Design review of the part built by this model. Coordinates are the model's own, in mm. A direction names the side the tool comes from. Coordinates: 2 decimals unless noted, no trailing zeros. Loops run counter-clockwise (first coordinate to the right, second up) from the corner with the lowest first, then second, coordinate; pieces in that order, holes last. Notation, with made-up numbers: M 55,-12.75 L 97,-12.75 A21 cw 97,-4.75 Z; hole C 80,76 d4. An arc over 180 degrees is marked long. Answer as a JSON object with one key per item and string values. Group by question number.
1. To check wall thickness, follow probe 1 along Z at (x, y) = (20.25, 0.8); probe 2 along X at (y, z) = (3.6, 2.5); probe 3 along Y at (x, z) = (-18, 11) (3 decimals). State the ranges of each line that lie inside material, in increasing order.
2. Machinability: for faces 1 (the flat face through (-14, 3.46, 6)), 2 (the cylindrical face through (-4.5, 0.9, 5.9)), 3 (the flat face through (-9.7, 3.9, 5.5)), 4 (the flat face through (8, 2.5, 3)), 5 (the flat face through (-9.7, 3.9, 1.5)), which of the approach directions +Z, -Z, +X, -X, +Y, -Y give a long, thin tool a straight path to every point of the face, cutting with its end or side? Answer none if there is none.
3. Consider section B-B (x = 13.5). State the section outline as (y, z) points (3 decimals), then the cut area to 3 significant figures.
4. Consider section A-A (x = 20.25). State the section outline as (y, z) points (3 decimals), then the cut area to 3 significant figures.
5. Consider section C-C (x = 3.5). State the section outline as (y, z) points.
6. Insertion check: pin 1 (0.6 mm diameter, centred on x = 25, z = 2.5, fed in from -Y); pin 2 (0.8 mm diameter, centred on x = -10, y = 4, fed in from +Z); pin 3 (2 mm diameter, centred on x = 13, y = 1.5, fed in from -Z); pin 4 (0.5 mm diameter, centred on x = -18.5, y = 4, fed in from -Z). Each pin has a flat end and moves straight along its axis. Give the tip position at first contact, or say it passes through.
Autodesk Inventor part; units mm, degrees
ref_plane "Work Plane1" through (-2.9282, 3.7996, 12.5) normal (0, 1, 0) x (1, 0, 0)
ref_plane "Work Plane2" through (0, 0, 1.5) normal (0, 0, -1) x (-1, 0, 0)
ref_plane "Work Plane4" through (0, 0, 0.45) normal (0, 0, -1) x (-1, 0, 0)
sketch "Sketch1" plane through (0, 0, 0) normal (0, 0, 1) x (1, 0, 0)
  arc A0 (-21.6, 0) -> (-23.4, 0) centre (-22.5, 0) ccw
  arc A1 (-15.975, 0) -> (-20.025, 0) centre (-18, 0) ccw
  arc A2 (-11.475, 0) -> (-15.525, 0) centre (-13.5, 0) ccw
  arc A3 (-6.975, 0) -> (-11.025, 0) centre (-9, 0) ccw
  arc A4 (-3.6, 0) -> (-5.4, 0) centre (-4.5, 0) ccw
  arc A5 (2.025, 0) -> (-2.025, 0) centre (0, 0) ccw
  arc A6 (6.525, 0) -> (2.475, 0) centre (4.5, 0) ccw
  arc A7 (11.025, 0) -> (6.975, 0) centre (9, 0) ccw
  arc A8 (15.525, 0) -> (11.475, 0) centre (13.5, 0) ccw
  arc A9 (18.875, 0) -> (17.125, 0) centre (18, 0) ccw
  arc A10 (23.375, 0) -> (21.625, 0) centre (22.5, 0) ccw
  line L0 (-25, 0) -> (-25, 1.5)
  line L1 (-25, 0) -> (25, 0)
  line L2 (25, 0) -> (25, 1.5)
  arc A11 (25, 1.5) -> (24, 2.5) centre (24, 1.5) ccw
  arc A12 (-24, 2.5) -> (-25, 1.5) centre (-24, 1.5) ccw
  line L3 (-8.467, 2.5) -> (24, 2.5)
  line L4 (-19.1661, 2.65) -> (-18.6985, 3.46)
  line L5 (-18.6985, 3.46) -> (-9.1945, 3.46)
  line L6 (-9.1945, 3.46) -> (-8.7268, 2.65)
  line L7 (-9.1945, 3.46) -> (-8.2592, 3.46) construction
  arc A13 (-8.7268, 2.65) -> (-8.467, 2.5) centre (-8.467, 2.8) ccw
  line L8 (-19.4259, 2.5) -> (-24, 2.5)
  arc A14 (-19.4259, 2.5) -> (-19.1661, 2.65) centre (-19.4259, 2.8) ccw
  line L9 (0, 0) -> (0, 12.7088) construction
  point P0 (-19.2527, 2.5)
  point P1 (-8.6402, 2.5)
  dimension "d1" = 1.8
  dimension "d2" = 4.5
  dimension "d3" = 4.5
  dimension "d4" = 4.5
  dimension "d5" = 4.5
  dimension "d6" = 4.5
  dimension "d7" = 4.5
  dimension "d8" = 4.5
  dimension "d9" = 4.5
  dimension "d10" = 4.5
  dimension "d11" = 4.5
  dimension "d12" = 4.05
  dimension "d13" = 4.05
  dimension "d14" = 4.05
  dimension "d15" = 1.8
  dimension "d16" = 4.05
  dimension "d17" = 4.05
  dimension "d18" = 4.05
  dimension "d19" = 4.05
  dimension "d20" = 1.75
  dimension "d21" = 1.75
  dimension "d22" = 2.5
  dimension "d23" = 50
  dimension "d24" = 1.5
  dimension "d25" = 1.5
  dimension "d26" = 1
  dimension "d27" = 1
  dimension "d29" = 120
  dimension "d32" = 9.504
  dimension "d33" = 60
  dimension "d67" = 0.96
  dimension "d68" = 0.3
  dimension "d69" = 0.3
  dimension "d70" = 33.467
  dimension "d71" = 5.5741
extrude "Extrusion1" add sketch "Sketch1" along normal blind 12 contours A0 L1 L0 A12 L8 A14 L4 L5 L6 A13 L3 A11 L2 A10 A9 A8 A7 A6 A5 A4 A3 A2 A1
sketch "Sketch2" plane through (0, 0, 12) normal (0, 0, 1) x (1, 0, 0)
  line L0 (-9.1945, 3.46) -> (-18.6985, 3.46)
  point P0 (0, 0)
  point P1 (-16.1965, 3.46)
  point P2 (-11.6965, 3.46)
  dimension "d39" = 4.5
  dimension "d40" = 2.502
hole "Hole1" at (-16.1965, 3.46, 12) at (-11.6965, 3.46, 12) direction (0, 0, -1) diameter 2 end through all
sketch "Sketch3" plane through (24, 2.5, 12) normal (0, 1, 0) x (1, 0, 0)
  line L0 (0.714, 6.4) -> (-32.467, 6.4)
  line L1 (-32.467, 6.4) -> (-32.467, 7)
  line L2 (-32.467, 7) -> (0.714, 7)
  line L3 (0.714, 7) -> (0.714, 6.4)
  line L4 (-32.467, 11) -> (0.714, 11)
  line L5 (0.714, 11) -> (0.714, 11.6)
  line L6 (0.714, 11.6) -> (-32.467, 11.6)
  line L7 (-32.467, 11.6) -> (-32.467, 11)
  line L8 (1, 12) -> (1, 0)
  line L9 (0, 12) -> (-32.467, 12)
  line L10 (-43.4259, 6.4) -> (-48.29, 6.4)
  line L11 (-48.29, 6.4) -> (-48.29, 7)
  line L12 (-48.29, 7) -> (-43.4259, 7)
  line L13 (-43.4259, 7) -> (-43.4259, 6.4)
  line L14 (-43.4259, 11.6) -> (-48.29, 11.6)
  line L15 (-48.29, 11.6) -> (-48.29, 11)
  line L16 (-48.29, 11) -> (-43.4259, 11)
  line L17 (-43.4259, 11) -> (-43.4259, 11.6)
  line L18 (-49, 12) -> (-49, 0)
  point P0 (-24, 12)
  point P1 (-32.5535, 12.5)
  point P2 (-32.467, 12)
  point P3 (-43.4259, 12)
  dimension "d48" = 0.286
  dimension "d49" = 0.286
  dimension "d50" = 0.6
  dimension "d51" = 0.6
  dimension "d57" = 0.4
  dimension "d58" = 4
  dimension "d79" = 0.71
extrude "Extrusion2" cut sketch "Sketch3" against normal blind 0.3
ref_plane "Work Plane1" through (-2.9282, 3.7996, 12.5) normal (0, 1, 0) x (1, 0, 0)
sketch "Sketch4" plane through (-2.9282, 2.5, 12.5) normal (0, 1, 0) x (1, 0, 0)
  line L0 (27.9282, 12.5495) -> (27.9282, 3.2148)
  line L1 (26.9282, 11.5) -> (-5.5388, 11.5)
  line L2 (27.9282, 12.5) -> (27.9282, 0.5)
  line L3 (-22.0718, 12.5) -> (-22.0718, 0.5)
  point P0 (2.9282, 12.5)
  point P1 (-17.8838, 9.5)
  point P2 (0.1157, 9.5)
  point P3 (23.1782, 9.5)
  dimension "d54" = 4.75
  dimension "d72" = 2
  dimension "d121" = 4.188
  dimension "d122" = 23.0625
hole "Hole2" at (-20.812, 2.5, 3) at (-2.8125, 2.5, 3) at (20.25, 2.5, 3) direction (0, -1, 0) diameter 1.5 end through all both
sketch "Sketch5" plane through (-8.467, 2.5, 12) normal (0, 1, 0) x (1, 0, 0)
  circle A0 centre (34.867, 2.0003) radius 2
  line L0 (32.467, 0) -> (33.467, 0)
  line L1 (33.467, 12) -> (33.467, 0)
  line L2 (33.467, 0) -> (33.467, 0.572)
  point P0 (8.467, 12)
  dimension "d73" = 4
  dimension "d75" = 1.4
  dimension "d76" = 0.572
extrude "Extrusion3" cut sketch "Sketch5" against normal blind 7.05
mirror "Mirror1" about plane through (0, 0, 0) normal (1, 0, 0) of "Extrusion3"
ref_plane "Work Plane2" through (0, 0, 1.5) normal (0, 0, -1) x (-1, 0, 0)
sketch "Sketch6" plane through (0, 0, 1.5) normal (0, 0, -1) x (-1, 0, 0)
  line L0 (8.7268, 2.65) -> (9.1945, 3.46)
  line L1 (9.1945, 3.46) -> (9.7718, 4.46)
  line L2 (9.1945, 3.46) -> (10.6965, 3.46)
  line L3 (9.7718, 4.46) -> (9.9768, 4.46)
  line L4 (9.9768, 4.46) -> (10.1968, 4.16)
  line L5 (10.1968, 4.16) -> (9.8968, 4.16)
  line L6 (9.8968, 4.16) -> (9.8968, 3.46)
  line L7 (9.1945, 3.46) -> (10.6965, 3.46)
  line L8 (9.8968, 3.46) -> (9.1945, 3.46)
  line L9 (12.6965, 3.46) -> (15.1965, 3.46)
  line L10 (13.9465, 3.46) -> (13.9465, 5.3261) construction
  line L11 (17.1965, 3.46) -> (18.6985, 3.46)
  line L12 (18.6985, 3.46) -> (18.1211, 4.46)
  line L13 (18.6985, 3.46) -> (19.8532, 3.46) construction
  line L14 (18.1211, 4.46) -> (17.9161, 4.46)
  line L15 (17.9161, 4.46) -> (17.6961, 4.16)
  line L16 (17.6961, 4.16) -> (17.9961, 4.16)
  line L17 (17.9961, 4.16) -> (17.9961, 3.46)
  line L18 (17.9961, 3.46) -> (18.6985, 3.46)
  point P0 (0, 0)
  dimension "d81" = 1
  dimension "d82" = 0.205
  dimension "d83" = 126.25
  dimension "d84" = 0.3
  dimension "d85" = 0.3
  dimension "d94" = 120
  dimension "d95" = 1
  dimension "d96" = 0.205
  dimension "d97" = 53.75
  dimension "d98" = 53.75
  dimension "d99" = 0.3
  dimension "d100" = 0.3
extrude "Extrusion4" add sketch "Sketch6" against normal blind 4
ref_plane "Work Plane4" through (0, 0, 0.45) normal (0, 0, -1) x (-1, 0, 0)
sketch "Sketch7" plane through (0, 0, 0.45) normal (0, 0, -1) x (-1, 0, 0)
  line L0 (24.9987, 1.55) -> (24.4667, 1.55)
  line L1 (25, 0) -> (20.025, 0)
  arc A0 (15.1965, 3.46) -> (17.1965, 3.46) centre (16.1965, 3.46) ccw
  line L2 (12.6965, 3.46) -> (15.1965, 3.46)
  arc A1 (10.6965, 3.46) -> (12.6965, 3.46) centre (11.6965, 3.46) ccw
  line L3 (9.1945, 3.46) -> (10.6965, 3.46)
  line L4 (8.7268, 2.65) -> (9.1945, 3.46)
  arc A2 (8.467, 2.5) -> (8.7268, 2.65) centre (8.467, 2.8) ccw
  line L5 (-24, 2.5) -> (8.467, 2.5)
  arc A3 (-24, 2.5) -> (-25, 1.5) centre (-24, 1.5) ccw
  line L6 (-25, 0) -> (-25, 1.5)
  line L7 (-23.375, 0) -> (-25, 0)
  arc A4 (-21.625, 0) -> (-23.375, 0) centre (-22.5, 0) ccw
  line L8 (-18.875, 0) -> (-21.625, 0)
  arc A5 (-17.125, 0) -> (-18.875, 0) centre (-18, 0) ccw
  line L9 (-15.525, 0) -> (-17.125, 0)
  arc A6 (-11.475, 0) -> (-15.525, 0) centre (-13.5, 0) ccw
  line L10 (-11.025, 0) -> (-11.475, 0)
  arc A7 (-6.975, 0) -> (-11.025, 0) centre (-9, 0) ccw
  line L11 (-6.525, 0) -> (-6.975, 0)
  arc A8 (-2.475, 0) -> (-6.525, 0) centre (-4.5, 0) ccw
  line L12 (-2.025, 0) -> (-2.475, 0)
  arc A9 (2.025, 0) -> (-2.025, 0) centre (0, 0) ccw
  line L13 (3.6, 0) -> (2.025, 0)
  arc A10 (5.4, 0) -> (3.6, 0) centre (4.5, 0) ccw
  line L14 (6.975, 0) -> (5.4, 0)
  arc A11 (11.025, 0) -> (6.975, 0) centre (9, 0) ccw
  line L15 (11.475, 0) -> (11.025, 0)
  arc A12 (15.525, 0) -> (11.475, 0) centre (13.5, 0) ccw
  line L16 (15.975, 0) -> (15.525, 0)
  arc A13 (20.025, 0) -> (15.975, 0) centre (18, 0) ccw
  line L17 (25, 0) -> (23.4, 0)
  line L18 (25, 1.5) -> (25, 0)
  arc A14 (25, 1.5) -> (24, 2.5) centre (24, 1.5) ccw
  line L19 (19.4259, 2.5) -> (24, 2.5)
  arc A15 (19.1661, 2.65) -> (19.4259, 2.5) centre (19.4259, 2.8) ccw
  line L20 (18.6985, 3.46) -> (19.1661, 2.65)
  line L21 (17.1965, 3.46) -> (18.6985, 3.46)
  line L22 (24.4667, 1.55) -> (24.124, 0.7504)
  line L23 (24.4667, 1.55) -> (25.3367, 1.55) construction
  line L24 (24.124, 0.7504) -> (24.4, 0.7504)
  line L25 (24.4, 0.7504) -> (24.4, 0)
  line L26 (24.4, 0) -> (25, 0)
  arc A16 (25, 1.5) -> (24, 2.5) centre (24, 1.5) ccw
  line L27 (25, 0) -> (25, 1.5)
  line L28 (21.6, 0) -> (20.025, 0)
  arc A17 (23.4, 0) -> (21.6, 0) centre (22.5, 0) ccw
  point P0 (0, 0)
  dimension "d102" = 1.55
  dimension "d103" = 0.532
  dimension "d104" = 113.2
  dimension "d105" = 0.87
  dimension "d106" = 0.276
extrude "Extrusion5" cut sketch "Sketch7" against normal blind 6.1 contours A14 L18 L1 L25 L24 L22 L0
sketch "Sketch8" plane through (0, 0, 12) normal (0, 0, 1) x (1, 0, 0)
  line L0 (-22, 0) -> (23, 0)
  line L1 (23, 0) -> (23, 0.175)
  line L2 (23, 0.175) -> (-22, 0.175)
  line L3 (-22, 0.175) -> (-22, 0)
  line L4 (25, 0) -> (25, 1.5)
  point P0 (0, 0)
  point P1 (21.625, 0)
  dimension "d109" = 0.175
  dimension "d110" = 45
  dimension "d111" = 2
extrude "Extrusion6" cut sketch "Sketch8" against normal through all
ref_plane "Work Plane5" through (0, 0, 0.75) normal (0, 0, -1) x (-1, 0, 0)
sketch "Sketch9" plane through (0, 0, 0.75) normal (0, 0, -1) x (-1, 0, 0)
  line L0 (24.9987, 1.55) -> (24.4667, 1.55)
  line L1 (25, 0) -> (24.25, 0)
  line L2 (25, 1.5) -> (25, 0)
  line L3 (24.4667, 1.55) -> (24.124, 0.7504)
  line L4 (24.4667, 1.55) -> (25.3367, 1.55) construction
  line L5 (24.124, 0.7504) -> (24.4, 0.7504)
  line L6 (24.4, 0.7504) -> (24.4, 0)
  line L7 (24.4, 0) -> (25, 0)
  line L8 (25, 0) -> (25, 1.5)
  line L9 (0, 0) -> (0, 5.6827) construction
  line L10 (-24.9987, 1.55) -> (-24.4667, 1.55)
  line L11 (-24.4, 0.7504) -> (-24.4, 0)
  line L12 (-25, 0.7504) -> (-25, 0)
  line L13 (-24.4, 0) -> (-25, 0)
  line L14 (-25, 0) -> (-25, 1.5)
  line L15 (-24.4667, 1.55) -> (-25.3367, 1.55) construction
  line L16 (-25, 0) -> (-24.25, 0)
  line L17 (-24.124, 0.7504) -> (-24.4, 0.7504)
  line L18 (-24.4667, 1.55) -> (-24.124, 0.7504)
  arc A0 (-24, 2.5) -> (-25, 1.5) centre (-24, 1.5) ccw
  arc A1 (-24.9987, 1.55) -> (-25, 1.5) centre (-24, 1.5) ccw
  point P0 (24.25, 0)
  point P1 (24, 1.5)
  point P2 (24, 1.5)
  point P3 (-24.25, 0)
  point P4 (-24, 1.5)
  point P5 (-24, 1.5)
  dimension "d115" = 0.532
  dimension "d116" = 113.2
  dimension "d117" = 0.87
  dimension "d118" = 0.276
extrude "Extrusion7" cut sketch "Sketch9" against normal blind 6.1
properties part number "3d_LM - Pinza 2" material "PA12 SLS 3D Print"
Findings below:
{
 "1": {"probe 1": "z = 0 to 2.25, 3.75 to 12", "probe 2": "x = -18.62 to -18, -9.9 to -9.28", "probe 3": "y = 2.025 to 3.46"},
 "2": {"face 1": "+Z, -Z, +Y", "face 2": "+Z, -Z, -Y", "face 3": "+Z, +X, -X, +Y", "face 4": "+Z, -Z, +X, +Y", "face 5": "-Z, +X, -X, +Y"},
 "3": {"outline": "M 2.025,0 L 2.5,0 L 2.5,0.4 L 2.2,0.4 L 2.2,1 L 2.5,1 L 2.5,5 L 2.2,5 L 2.2,5.6 L 2.5,5.6 L 2.5,12 L 2.025,12 Z", "area": "5.34 mm^2"},
 "4": {"outline": "M 0.175,0 L 2.5,0 L 2.5,0.4 L 2.2,0.4 L 2.2,1 L 2.5,1 L 2.5,2.25 L 0.175,2.25 Z; M 0.175,3.75 L 2.5,3.75 L 2.5,5 L 2.2,5 L 2.2,5.6 L 2.5,5.6 L 2.5,12 L 0.175,12 Z", "area": "24.1 mm^2"},
 "5": {"outline": "M 1.76,0 L 2.5,0 L 2.5,0.4 L 2.2,0.4 L 2.2,1 L 2.5,1 L 2.5,5 L 2.2,5 L 2.2,5.6 L 2.5,5.6 L 2.5,12 L 1.76,12 Z"},
 "6": {"pin 1": "stops at y = 1.55", "pin 2": "stops at z = 5.5", "pin 3": "stops at z = 0", "pin 4": "stops at z = 1.5"}
}
